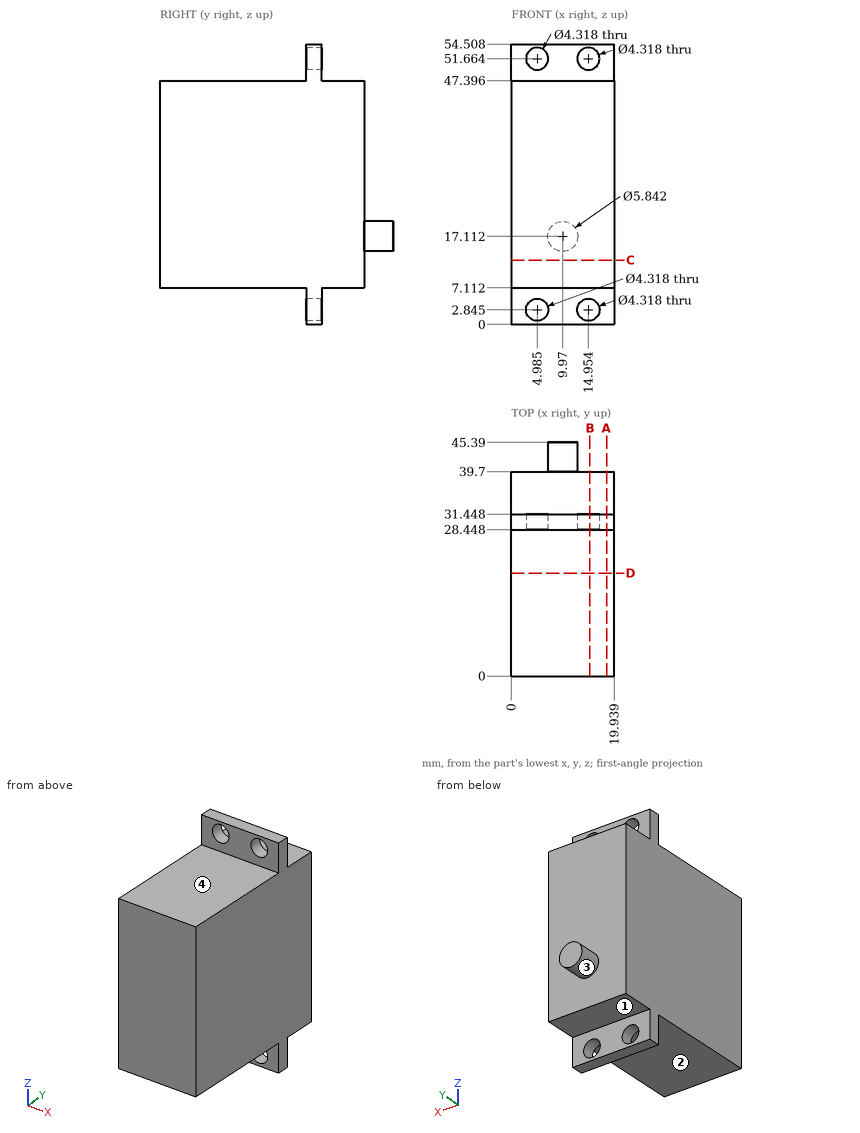
Source: three-view drawing plus pictorial views. Frame: mm from the lowest corner of the part. A direction names the side the tool comes from. Give positions to 0.01 mm unless a question says otherwise; leave off trailing zeros. Order: outer loops, then holes, each group sorted by start corner. A loop starts at its lowest first (then second) coordinate and runs counter-clockwise, first axis right, second up. Notation, with made-up numbers: (56.25, 75) -> (71.25, 75) arc R22 cw to (71.25, 101) -> close; hole circle Ø1 at (-10, 43.5). An arc over 180 degrees is marked (long way). Put each result on its own line as item: value.
Q1. Material intervals for L1, parallel to Z at x = 6, y = 30; L2, parallel to Z at x = 16.5, y = 31.5; L3, parallel to Y at x = 16, z = 29.5, sorted ascending.
Here are the results:
L1: z = 0 to 0.94, 4.75 to 49.76, 53.57 to 54.51
L2: z = 7.11 to 47.4
L3: y = 0 to 39.7
Q2. Section C-C, the plane z = 12.5. Return loops of the section in (x, y).
Here are the results:
outline: (0, 0) -> (19.94, 0) -> (19.94, 39.7) -> (0, 39.7) -> close
Q3. Section A-A, the plane x = 18.5. Return loops of the section in (y, z), then the cut area to 3 significant figures.
Here are the results:
outline: (0, 7.11) -> (28.45, 7.11) -> (28.45, 0) -> (31.45, 0) -> (31.45, 7.11) -> (39.7, 7.11) -> (39.7, 47.4) -> (31.45, 47.4) -> (31.45, 54.51) -> (28.45, 54.51) -> (28.45, 47.4) -> (0, 47.4) -> close
area: 1,640 mm^2
Q4. Section D-D, the plane y = 20. Return loops of the section in (x, z).
Here are the results:
outline: (0, 7.11) -> (19.94, 7.11) -> (19.94, 47.4) -> (0, 47.4) -> close
Q5. Reachability of the marked faces 1, 2, 3 and 4 from +Z, -Z, +X, -X, +Y, -Y: full face, straight path, thin tool, end or side. Return the list, or none.
Here are the results:
face 1: -Z, +X, -X, +Y
face 2: -Z, +X, -X, -Y
face 3: +Y
face 4: +Z, +X, -X, -Y
Q6. Section B-B, the plane x = 15.25. Return loops of the section in (y, z) (1 decimal).
Here are the results:
outline: (0, 7.1) -> (28.4, 7.1) -> (28.4, 5) -> (31.4, 5) -> (31.4, 7.1) -> (39.7, 7.1) -> (39.7, 47.4) -> (31.4, 47.4) -> (31.4, 49.5) -> (28.4, 49.5) -> (28.4, 47.4) -> (0, 47.4) -> close; (28.4, 0) -> (31.4, 0) -> (31.4, 0.7) -> (28.4, 0.7) -> close; (28.4, 53.8) -> (31.4, 53.8) -> (31.4, 54.5) -> (28.4, 54.5) -> close
Q7. Pin query (flat end, axial travel): pin 1 (3.5 mm diameter, centred on x = 7, z = 51.5, fed in from +Y); pin 2 (8 mm diameter, centred on x = 3.5, z = 35, fed in from +Y); pin 3 (3.5 mm diameter, centred on x = 8.5, z = 51, fed in from -Y); pin 4 (2.5 mm diameter, centred on x = 4.98, z = 2.84, fed in from -Y). Return the tip coordinate at first contact, or that it passes through.
Here are the results:
pin 1: stops at y = 31.45
pin 2: stops at y = 39.7
pin 3: stops at y = 28.45
pin 4: passes through
